The model under review builds one solid part; all positions refer to its coordinate system, in mm. A direction names the side the tool comes from. Coordinates: 2 decimals unless noted, no trailing zeros. Write each loop counter-clockwise with the first axis right and the second up, starting at its lowest first coordinate (ties: lowest second). Pieces come first, ordered by that corner, then holes. Notation, with made-up numbers: (14, 30.5) - (24, 30.5) arc R17 ccw to (24, 46.5) - close; hole circle Ø7 at (89, -4.5). An arc over 180 degrees is marked (long way). Return JSON: item names as keys, results as strings. Group by question number.
(1) We need section C-C on z = 35.5. State the section outline as (x, y) points, then the cut area to 3 significant figures.
(2) We need section D-D on z = 22. State the section outline as (x, y) points, then the cut area to 3 significant figures.
(3) For pin 1 Ø4 at (y, z) = (8.5, -14.5) entering from -X; pin 2 Ø7.5 at (x, z) = (-11, -10) entering from -Y; pin 3 Ø5 at (y, z) = (-8, 30.5) entering from +X, all flat-tipped, find the tip position at first contact; note any pin that passes through.
(4) Tool access review of faces 5 (the face through (7, 14.335, 26)), 6 (the face through (20, -2.645, 32)), 7 (the face through (-1, 16.531, -13)), 8 (the face through (-1, -16.531, -13)): name each direction out of +Z, -Z, +X, -X, +Y, -Y from which nothing blocks a thin tool from reaching the whole face with its end or side.
(5) We need section A-A on x = -12. State the section outline as (y, z) points.
(6) Draft analysis for pull direction Z (two halves, no side actions). For faces 1 (the face through (-11, 0, 50.8)), 2 (the face through (-1, 26.67, 25)), 3 (the face through (20, -10, 26.67)), 4 (the face through (0, -10, 32)), state which applies: released by +Z, released by -Z, zero draft, split by the parting line, or undercut.
(7) To check wall thickness, follow L1, parallel to Z at x = 8.5, y = -12.5; L2, parallel to Y at x = 33.5, z = 27.5; L3, parallel to Z at x = 40.5, y = -4. State the ranges of each line that lie inside material, in increasing order. Write a range as from..to.
(8) We need section B-B on y = 7. State the section outline as (x, z) points, then the cut area to 3 significant figures.
```python
from build123d import *

# Parameters (mm, degrees)
F0_W      = 96.10016644
F0_H      = 53.3400028944
F1_DEPTH  = 50.8
F2_W      = 73.1771886349
F2_H      = 33.0619849265
F3_DEPTH  = 25.4
F4_W      = 13.6656195391
F4_H      = 10.1390071213
F5_DEPTH  = 48.05108322
F7_DEPTH  = 53.3410028944
F9_DEPTH  = 43.18
F11_DEPTH = 25.4


with BuildPart() as f1:
    # F0 (on Top) → F1 (new body)
    with BuildSketch(Plane.XY):
        Rectangle(F0_W, F0_H)
    extrude(amount=F1_DEPTH)

    # F2 (on Top) → F3 (join)
    with BuildSketch(Plane.XY):
        Rectangle(F2_W, F2_H)
    extrude(amount=-F3_DEPTH)

    # F4 (on Right) → F5 (cut, through all)
    with BuildSketch(Plane.YZ):
        with Locations((-9.4777684426, 31.7395050079)):
            Rectangle(F4_W, F4_H)
    extrude(amount=F5_DEPTH, mode=Mode.SUBTRACT)

    # F6 (on face) → F7 (cut, through all)
    with BuildSketch(Plane(origin=(0, 26.6700014472, 0), x_dir=(-1, 0, 0), z_dir=(0, 1, 0))):
        Polygon((-48.05008322, 50.8), (-48.05008322, 14.7308725864), (-26.2037906796, 50.8), align=None)
    extrude(amount=-F7_DEPTH, mode=Mode.SUBTRACT)

    # F8 (on face) → F9 (cut)
    with BuildSketch(Plane(origin=(41.6815353707, 0, 25.2456069924), x_dir=(0, 1, 0), z_dir=(0.8553426921, 0, 0.5180626207))):
        Polygon((11.9023136795, 5.7883295231), (9.2573547736, 3.2114295755), (14.6670065658, -2.3410974829), (22.4821474403, -2.3410974829), (22.4821474403, 5.7883295231), align=None)
    extrude(amount=-F9_DEPTH, mode=Mode.SUBTRACT)

    # F10 (on face) → F11 (cut)
    with BuildSketch(Plane(origin=(-2.9987171623, 0, 4.9510053573), x_dir=(0.8553426921, 0, 0.5180626207), z_dir=(0.5180626207, 0, -0.8553426921))):
        Polygon((29.4420253485, -19.3029493093), (28.2331872731, -14.3353175372), (10.6222741306, -14.3353175372), (10.6222741306, -19.3029493093), align=None)
    extrude(amount=-F11_DEPTH, mode=Mode.SUBTRACT)


solid = f1.part
```
Ans:
{
 "1": {"outline": "(-48.05, -26.67) - (35.47, -26.67) - (35.47, -16.31) - (0, -16.31) - (0, -2.64) - (35.47, -2.64) - (35.47, 26.67) - (-48.05, 26.67) - close; hole (-1.59, 14.34) - (11.51, 14.34) - (12.92, 19.3) - (-1.59, 19.3) - close", "area": "3,900 mm²"},
 "2": {"outline": "(-48.05, -26.67) - (43.65, -26.67) - (43.65, 26.67) - (-48.05, 26.67) - close; hole (-0.91, 14.34) - (19.68, 14.34) - (21.1, 19.3) - (-0.91, 19.3) - close; hole (25.15, 11.9) - (30.12, 9.26) - (40.84, 14.67) - (40.84, 22.48) - (25.15, 22.48) - close", "area": "4,610 mm²"},
 "3": {"pin 1": "x = -36.59", "pin 2": "y = -16.53", "pin 3": "x = 0"},
 "4": {"face 5": "none", "face 6": "+X", "face 7": "-Z, +X, -X, +Y", "face 8": "-Z, +X, -X, -Y"},
 "5": {"outline": "(-26.67, 0) - (-16.53, 0) - (-16.53, -25.4) - (16.53, -25.4) - (16.53, 0) - (26.67, 0) - (26.67, 50.8) - (-26.67, 50.8) - close"},
 "6": {"face 1": "released by +Z", "face 2": "zero draft", "face 3": "undercut", "face 4": "undercut"},
 "7": {"L1": "-25.4..26.67, 36.81..50.8", "L2": "-26.67..-16.31, -2.64..26.67", "L3": "0..26.67"},
 "8": {"outline": "(-48.05, 0) - (-36.59, 0) - (-36.59, -25.4) - (36.59, -25.4) - (36.59, 0) - (48.05, 0) - (48.05, 14.73) - (26.2, 50.8) - (-48.05, 50.8) - close", "area": "6,350 mm²"}
}
